Build history of the part. All positions in model axes, mm. Give positions to 0.01 mm unless a question says otherwise; leave off trailing zeros. Order: outer loops, then holes, each group sorted by start corner. A loop starts at its lowest first (then second) coordinate and runs counter-clockwise, first axis right, second up. Notation, with made-up numbers: (20.25, -20) - (75.25, -20) arc R34 cw to (75.25, 11) - close; hole circle Ø5 at (64, -9.5). An arc over 180 degrees is marked (long way). Use a Markdown table: item, result. Add a question column.
(1) Wall check: line 1 (X direction, y = 26, z = 2.1); line 2 (Y direction, x = 0, z = 1.95); line 3 (Y direction, x = 17, z = 2.65). Give the ranges that are in metal, low to high.
(2) Mould opens along X. For faces 1 (the face through (16.94, -39.41, 2.96)), 2 (the face through (16.94, 37.59, 2.96)), 3 (the face through (-10.3, 46.37, 2.96)), 4 (the face through (10, 1, 6)) say: +X half, -X half, draft (parallel to the pull), parting line (faces both ways), or undercut.
(3) Slice it at A-A (y = 0). Write the cut outline in (x, z).
(4) Slice it at C-C (z = 3.15). Count the separate pieces of the cut face and the enclosed holes in it, then the cut area to 3 significant figures.
(5) Slice it at D-D (y = 26). Write the cut outline in (x, z), then the cut area to 3 significant figures.
(6) Flat gauge pins, fed straight in: pin 1 (2 mm diameter, centred on y = -4.5, z = 0.5, fed in from -X); pin 2 (3 mm diameter, centred on x = -31, z = 1, fed in from +Y); pin 3 (1.5 mm diameter, centred on x = 24.5, z = 1.5, fed in from -Y). Where does each tip first touch, or does it go through?
Autodesk Inventor part; units mm, degrees
ref_plane "YZ Plane" through (0, 0, 0) normal (1, 0, 0) x (0, 1, 0)
ref_plane "XZ Plane" through (0, 0, 0) normal (0, 1, 0) x (-1, 0, 0)
ref_plane "XY Plane" through (0, 0, 0) normal (0, 0, 1) x (1, 0, 0)
sketch "Sketch1" plane through (0, 0, 0) normal (0, 0, 1) x (1, 0, 0)
  circle A0 centre (0, 0) radius 47.5
  dimension "d0" = 95
extrude "Extrusion1" add sketch "Sketch1" along normal blind 6
sketch "Sketch12" plane through (0, 0, 0) normal (0, 0, -1) x (-1, 0, 0)
  line L0 (15.75, 36.5709) -> (15.75, -44.8128)
  circle A0 centre (0, 0) radius 47.5
  line L1 (-15.75, 36.5709) -> (-15.75, -44.8128)
  line L2 (-15.75, 36.5709) -> (-15.75, 44.8128)
  line L3 (15.75, 36.5709) -> (15.75, 45.8997)
  line L4 (0, 0) -> (0, 26)
  line L5 (0, 26) -> (0, -26)
  line L6 (0, -26) -> (15.75, -26)
  line L7 (-15.75, -26) -> (0, -26)
  line L8 (0, 26) -> (15.75, 26)
  line L9 (-15.75, 26) -> (0, 26)
  circle A1 centre (-15.75, 26) radius 1.5
  circle A2 centre (15.75, 26) radius 1.5
  circle A3 centre (15.75, -26) radius 1.5
  circle A4 centre (-15.75, -26) radius 1.5
  line L10 (-15.75, 26) -> (-15.75, 38.5)
  line L11 (-15.75, 38.5) -> (15.75, 38.5)
  circle A5 centre (-15.75, 38.5) radius 1.5
  circle A6 centre (15.75, 38.5) radius 1.5
  line L12 (-15.75, -26) -> (-15.75, -38.5)
  line L13 (-15.75, -38.5) -> (15.75, -38.5)
  circle A7 centre (15.75, -38.5) radius 1.5
  circle A8 centre (-15.75, -38.5) radius 1.5
extrude "Extrusion2" cut sketch "Sketch12" against normal blind 10 contours A2 L0 | L0 L8 A2 | A6 L11 L3 | L3 A6 | L0 A2 L8 | L11 A6 L3 | A5 L2 L11 | L11 L2 A5 | A3 L0 | L0 L6 A3 | A1 L1 L9 | L9 L1 A1 | L2 A5 | L0 A3 L6 | L1 A1 | A4 L1 L7 | L7 L1 A4 | L1 A4 | A7 L0 | L0 L13 A7 | A7 L13 L0 | A8 L1 | L1 L13 A8 | A8 L13 L1
sketch "Sketch14" plane through (0, 0, 6) normal (0, 0, 1) x (1, 0, 0)
  point P0 (0, 0)
sketch "Sketch15" plane through (0, 0, 6) normal (0, 0, 1) x (1, 0, 0)
  circle A0 centre (0, 0) radius 1.5
  dimension "d22" = 3
extrude "Extrusion4" cut sketch "Sketch15" against normal blind 10
properties part number "podstawa"
Solution:
| question | item | result |
|---|---|---|
| 1 | line 1 | -39.75 to -17.25, -14.25 to 14.25, 17.25 to 39.75 |
| 1 | line 2 | -47.5 to -1.5, 1.5 to 47.5 |
| 1 | line 3 | -44.35 to -39.33, -37.67 to -26.83, -25.17 to 25.17, 26.83 to 37.67, 39.33 to 44.35 |
| 2 | face 1 | undercut |
| 2 | face 2 | undercut |
| 2 | face 3 | parting line |
| 2 | face 4 | draft |
| 3 | outline | (-47.5, 0) - (-1.5, 0) - (-1.5, 6) - (-47.5, 6) - close; (1.5, 0) - (47.5, 0) - (47.5, 6) - (1.5, 6) - close |
| 4 | separate pieces | 1 |
| 4 | enclosed holes | 9 |
| 4 | area | 7,020 mm2 |
| 5 | outline | (-39.75, 0) - (-17.25, 0) - (-17.25, 6) - (-39.75, 6) - close; (-14.25, 0) - (14.25, 0) - (14.25, 6) - (-14.25, 6) - close; (17.25, 0) - (39.75, 0) - (39.75, 6) - (17.25, 6) - close |
| 5 | area | 441 mm2 |
| 6 | pin 1 | x = -47.37 |
| 6 | pin 2 | y = 37.23 |
| 6 | pin 3 | y = -41.14 |
